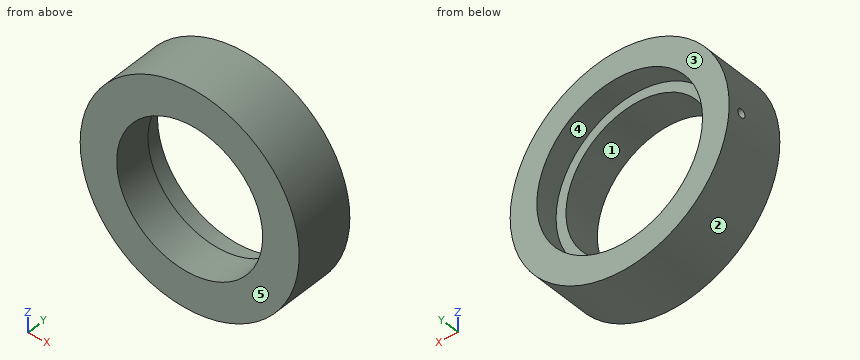
from build123d import *

# Parameters (mm, degrees)
F0_R     = 45
F0_R_2   = 30
F1_DEPTH = 25
F2_R     = 34.05
F3_DEPTH = 9.5
F5_R     = 1.75
F6_DEPTH = 25


with BuildPart() as f1:
    # F0 (on Front) → F1 (new body)
    with BuildSketch(Plane.XZ):
        Circle(F0_R)
        Circle(F0_R_2, mode=Mode.SUBTRACT)
    extrude(amount=F1_DEPTH)

    # F2 (on face) → F3 (cut)
    with BuildSketch(Plane(origin=(0, 0, 0), x_dir=(-1, 0, 0), z_dir=(0, 1, 0))):
        Circle(F2_R)
    extrude(amount=-F3_DEPTH, mode=Mode.SUBTRACT)

    # F5 (on offset) → F6 (cut)
    with BuildSketch(Plane.YZ.offset(-45)):
        with Locations((-6, 0)):
            Circle(F5_R)
    extrude(amount=F6_DEPTH, mode=Mode.SUBTRACT)


solid = f1.part
Work out the finished part from the listing and answer in its coordinate system (mm). Face numbers are marked on the shaded views. A direction names the side the tool comes from. Round coordinates to 2 decimals unless told otherwise and drop trailing zeros. Write each loop counter-clockwise with the first axis right and the second up, starting at its lowest first coordinate (ties: lowest second). Pieces come first, ordered by that corner, then holes. Notation, with made-up numbers: (-10, -39) - (0, -39) arc R10 ccw to (0, -35) - close; hole circle Ø4 at (-13, 80). An arc over 180 degrees is marked (long way). Answer in a Markdown table with one row per item. Add a question column.
1. A cutting plane is placed at A-A, the plane z = 0. Determine the outline of the cut face in (x, y), and give its area (3 significant figures).
2. A cutting plane is placed at B-B, the plane x = 0. Determine the outline of the cut face in (y, z), and give its area (3 significant figures).
3. The mould has two halves that part along Z. Classify the marked faces 1, 2 and 3: +Z half, -Z half, draft (parallel to the pull), parting line (faces both ways), or undercut.
4. A cutting plane is placed at D-D, the plane y = -13.25. Determine the outline of the cut face in (x, z).
5. A cutting plane is placed at C-C, the plane z = -17. Determine the outline of the cut face in (x, y), and give its area (3 significant figures).
6. Given pin 1 (12 mm diameter, centred on y = -2.5, z = -2, fed in from -X); pin 2 (2 mm diameter, centred on y = -17.5, z = 4, fed in from -X); pin 3 (3 mm diameter, centred on y = -20, z = -24.5, fed in from -X); pin 4 (4 mm diameter, centred on x = 17, y = -8, fed in from +Z), each flat-ended and moving along its own axis, determine where each tip first touches the part or whether it passes through.
7. For the marked faces 4 and 5, determine the directions among +Z, -Z, +X, -X, +Y, -Y from which every point of the face is accessible in a straight line to the end or side of a thin tool.
8. Find the intervals of material crossed by line 1 along Z through (x, y) = (0, -19.75); line 2 along Z through (x, y) = (0, -6.5), in increasing order. Write a range as from..to.
Worked out:
| question | item | result |
|---|---|---|
| 1 | outline | (-45, -25) - (-30, -25) - (-30, -9.5) - (-34.05, -9.5) - (-34.05, -7.75) - (-45, -7.75) - close; (-45, -4.25) - (-34.05, -4.25) - (-34.05, 0) - (-45, 0) - close; (30, -25) - (45, -25) - (45, 0) - (34.05, 0) - (34.05, -9.5) - (30, -9.5) - close |
| 1 | area | 635 mm^2 |
| 2 | outline | (-25, -45) - (0, -45) - (0, -34.05) - (-9.5, -34.05) - (-9.5, -30) - (-25, -30) - close; (-25, 30) - (-9.5, 30) - (-9.5, 34.05) - (0, 34.05) - (0, 45) - (-25, 45) - close |
| 2 | area | 673 mm^2 |
| 3 | face 1 | undercut |
| 3 | face 2 | parting line |
| 3 | face 3 | draft |
| 4 | outline | circle Ø90 at (0, 0); hole circle Ø60 at (0, 0) |
| 5 | outline | (-41.67, -25) - (-24.72, -25) - (-24.72, -9.5) - (-29.5, -9.5) - (-29.5, 0) - (-41.67, 0) - close; (24.72, -25) - (41.67, -25) - (41.67, 0) - (29.5, 0) - (29.5, -9.5) - (24.72, -9.5) - close |
| 5 | area | 756 mm^2 |
| 6 | pin 1 | x = -45 |
| 6 | pin 2 | x = -44.9 |
| 6 | pin 3 | x = -38.68 |
| 6 | pin 4 | z = 42.43 |
| 7 | face 4 | +Y |
| 7 | face 5 | +Z, -Z, +X, -X, -Y |
| 8 | line 1 | -45..-30, 30..45 |
| 8 | line 2 | -45..-34.05, 34.05..45 |
